from build123d import *

# Parameters (mm, degrees)
SKETCH_1_W          = 70
SKETCH_1_H          = 40
EXTRUDE_1_DEPTH     = 1
SKETCH_2_R          = 3
CUT_EXTRUDE_1_DEPTH = 10
SKETCH_4_W          = 55
SKETCH_4_H          = 36
EXTRUDE_2_DEPTH     = 1.5
EXTRUDE_START       = -40
SKETCH_4_2_W        = 55
SKETCH_4_2_H        = 36
EXTRUDE_3_DEPTH     = 1.5
SKETCH_5_R          = 1.5
CUT_EXTRUDE_2_DEPTH = 41


with BuildPart() as part:
    # 草图1 → 凸台-拉伸1 (new body)
    with BuildSketch(Plane.XY):
        Rectangle(SKETCH_1_W, SKETCH_1_H)
    extrude(amount=EXTRUDE_1_DEPTH)

    # 草图2 → 切除-拉伸1 (cut)
    with BuildSketch(Plane.XY.offset(1)):
        with Locations((-25.5, 0)):
            Circle(SKETCH_2_R)
        with Locations((25.5, 0)):
            Circle(SKETCH_2_R)
    extrude(amount=-CUT_EXTRUDE_1_DEPTH, mode=Mode.SUBTRACT)

    # 草图4 → 凸台-拉伸2 (add)
    with BuildSketch(Plane(origin=(0, 20, 0), x_dir=(1, 0, 0), z_dir=(0, 1, 0))):
        with Locations((0, 17)):
            Rectangle(SKETCH_4_W, SKETCH_4_H)
    extrude(amount=-EXTRUDE_2_DEPTH)

    # 草图4<2> → 凸台-拉伸3 (add)
    with BuildSketch(Plane(origin=(0, 20, 0), x_dir=(1, 0, 0), z_dir=(0, 1, 0)).offset(EXTRUDE_START)):
        with Locations((0, 17)):
            Rectangle(SKETCH_4_2_W, SKETCH_4_2_H)
    extrude(amount=EXTRUDE_3_DEPTH)

    # 草图5 → 切除-拉伸2 (cut, through all)
    with BuildSketch(Plane(origin=(0, 20, 0), x_dir=(1, 0, 0), z_dir=(0, 1, 0))):
        with Locations((-14.5, 22.5)):
            Circle(SKETCH_5_R)
        with Locations((14.5, 22.5)):
            Circle(SKETCH_5_R)
    extrude(amount=-CUT_EXTRUDE_2_DEPTH, mode=Mode.SUBTRACT)


solid = part.part
Design review of the part built by this model. Coordinates are the model's own, in mm. A direction names the side the tool comes from. Coordinates: 2 decimals unless noted, no trailing zeros. Loops run counter-clockwise (first coordinate to the right, second up) from the corner with the lowest first, then second, coordinate; pieces in that order, holes last. Notation, with made-up numbers: (9.5, -18.75) - (37.5, -18.75) arc R14 cw to (37.5, -8.75) - close; hole circle Ø6 at (78, 79.25). An arc over 180 degrees is marked (long way). Use CSV: the item, a comma, the result in double quotes. Start each with the question number.
1. Mouldability with a two-part tool opening along Z and no side actions: class faces 4 (the cylindrical face through (-15.61, -19.24, -23.51)), 5 (the flat face through (0, -18.5, -18)), 6 (the flat face through (0, 0, 1)), 7 (the cylindrical face through (13.39, -19.24, -23.51)) as released by +Z, released by -Z, zero draft, split by the parting line, or undercut.
2. Clearance check with flat-ended pins moving along their axes: pin 1 (1.2 mm diameter, centred on y = 19, z = -24, fed in from +X); pin 2 (2.5 mm diameter, centred on x = -14.5, z = -22.5, fed in from +Y); pin 3 (10 mm diameter, centred on x = 10.5, y = -3, fed in from -Z). State where each tip first meets the part, or that it passes through.
3. Add section A-A on y = 0. Give the boundary of the cut face in (x, z), plus the area to 3 significant figures.
4. Add section D-D on x = 14.5. Give the boundary of the cut face in (y, z).
5. For faces 1 (the flat face through (-27.5, -19, -17)), 2 (the flat face through (27.5, -19, -17)), 3 (the flat face through (0, 18.5, -18)), list the 3-axis set-ups (+Z, -Z, +X, -X, +Y, -Y) from which the entire face can be reached by the end or side of a thin tool; tool diameter is ignored.
6. Add section C-C on z = -17. Give the boundary of the cut face in (x, y), plus the area to 3 significant figures.
7. Add section B-B on x = -25.5. Give the boundary of the cut face in (y, z), plus the area to 3 significant figures.
8. To check wall thickness, follow probe 1 along Y at (x, z) = (-20, -2.5); probe 2 along X at (y, z) = (19.25, -22.5); probe 3 along Z at (x, y) = (-14.5, -19.2). State the ranges of each line that lie inside material, in increasing order.
Resolved:
1,face 4,"undercut"
1,face 5,"zero draft"
1,face 6,"released by +Z"
1,face 7,"undercut"
2,pin 1,"x = 27.5"
2,pin 2,"through"
2,pin 3,"z = 0"
3,outline,"(-35, 0) - (-28.5, 0) - (-28.5, 1) - (-35, 1) - close; (-22.5, 0) - (22.5, 0) - (22.5, 1) - (-22.5, 1) - close; (28.5, 0) - (35, 0) - (35, 1) - (28.5, 1) - close"
3,area,"58.0 mm2"
4,outline,"(-20, -35) - (-18.5, -35) - (-18.5, -24) - (-20, -24) - close; (-20, -21) - (-18.5, -21) - (-18.5, 0) - (18.5, 0) - (18.5, -21) - (20, -21) - (20, 1) - (-20, 1) - close; (18.5, -35) - (20, -35) - (20, -24) - (18.5, -24) - close"
5,face 1,"-Z, -X, +Y, -Y"
5,face 2,"-Z, +X, +Y, -Y"
5,face 3,"-Z, +X, -X"
6,outline,"(-27.5, -20) - (27.5, -20) - (27.5, -18.5) - (-27.5, -18.5) - close; (-27.5, 18.5) - (27.5, 18.5) - (27.5, 20) - (-27.5, 20) - close"
6,area,"165 mm2"
7,outline,"(-20, -35) - (-18.5, -35) - (-18.5, 0) - (-3, 0) - (-3, 1) - (-20, 1) - close; (3, 0) - (18.5, 0) - (18.5, -35) - (20, -35) - (20, 1) - (3, 1) - close"
7,area,"139 mm2"
8,probe 1,"-20 to -18.5, 18.5 to 20"
8,probe 2,"-27.5 to -16, -13 to 13, 16 to 27.5"
8,probe 3,"-35 to -24, -21 to 1"
